Solid Edge part; units mm, degrees
sketch "Sketch1" plane through (0, 0, 0) normal (0, -1, 0) x (1, 0, 0)
  line L0 (-100, 125) -> (100, 125)
  line L1 (100, 125) -> (100, -125)
  line L2 (100, -125) -> (-100, -125)
  line L3 (-100, -125) -> (-100, 125)
  dimension "D1" = 100
  dimension "D2" = 100
extrude "Protrusion1" add sketch "Sketch1" along normal mid plane 6
sketch "Sketch2" plane through (0, -3, 0) normal (0, -1, 0) x (1, 0, 0)
  line L0 (-30, 55) -> (30, 55)
  line L1 (30, 55) -> (30, -5)
  line L2 (30, -5) -> (-30, -5)
  line L3 (-30, -5) -> (-30, 55)
  dimension "D1" = 30
  dimension "D2" = 30
extrude "Ausprägung_2" add sketch "Sketch2" along normal blind 1
hole "Bohrung_1" at (20, -4, 45) direction (0, 1, 0) diameter 8 end up to next
hole "Hole1" at (0, -4, 5) direction (0, 1, 0) diameter 8 end up to next
hole "Hole2" at (-20, -4, 45) direction (0, 1, 0) diameter 8 end up to next
sketch "Sketch3" plane through (0, -3, 0) normal (0, -1, 0) x (1, 0, 0)
  line L0 (-80, -125) -> (0, -45)
  line L1 (0, -45) -> (80, -125)
  line L2 (-80, -125) -> (80, -125)
  dimension "D1" = 80
extrude "Ausschnitt_1" cut sketch "Sketch3" against normal blind 146.05
sketch "Sketch4" plane through (0, -3, 0) normal (0, -1, 0) x (1, 0, 0)
  line L0 (-100, -105) -> (-30, -35)
  line L1 (-30, -35) -> (-30, -5)
  line L2 (-30, -5) -> (-30, 55)
  line L3 (-30, 55) -> (-100, 55)
  line L4 (-100, 55) -> (-100, -105)
  dimension "D1" = 100
extrude "Ausschnitt_2" cut sketch "Sketch4" against normal blind 200.025
sketch "Sketch5" plane through (0, -3, 0) normal (0, -1, 0) x (1, 0, 0)
  line L0 (100, -105) -> (30, -35)
  line L1 (30, -35) -> (30, -5)
  line L2 (30, -5) -> (30, 55)
  line L3 (30, 55) -> (100, 55)
  line L4 (100, 55) -> (100, -105)
extrude "Ausschnitt_3" cut sketch "Sketch5" against normal blind 184.15
sketch "Sketch6" plane through (0, -3, 90) normal (0, -1, 0) x (1, 0, 0)
  line L0 (-40, 35) -> (0, -5)
  line L1 (0, -5) -> (40, 35)
  line L2 (40, 35) -> (-40, 35)
  dimension "D1" = 40
extrude "Ausschnitt_4" cut sketch "Sketch6" against normal blind 88.9
sketch "Sketch7" plane through (0, -3, 90) normal (0, -1, 0) x (1, 0, 0)
  line L0 (-75.3553, 35) -> (-30, -10.3553)
  line L1 (-30, -10.3553) -> (-30, -35)
  line L2 (-30, -35) -> (-100, -35)
  line L3 (-100, -35) -> (-100, 35)
  line L4 (-100, 35) -> (-75.3553, 35)
  dimension "D1" = 30
extrude "Ausschnitt_5" cut sketch "Sketch7" against normal blind 38.1
sketch "Sketch8" plane through (12.3223, -3, 90) normal (0, -1, 0) x (1, 0, 0)
  line L0 (63.033, 35) -> (17.6777, -10.3553)
  line L1 (17.6777, -10.3553) -> (17.6777, -35)
  line L2 (17.6777, -35) -> (87.6777, -35)
  line L3 (87.6777, -35) -> (87.6777, 35)
  line L4 (87.6777, 35) -> (63.033, 35)
  dimension "D1" = 17.6777
extrude "Ausschnitt_6" cut sketch "Sketch8" against normal blind 104.775
sketch "Sketch9" plane through (0, -3, 90) normal (0, -1, 0) x (1, 0, 0)
  line L0 (-40, 35) -> (-57.6777, 17.3223)
  line L1 (-57.6777, 17.3223) -> (-75.3553, 35)
  line L2 (-75.3553, 35) -> (-40, 35)
extrude "Ausschnitt_7" cut sketch "Sketch9" against normal blind 63.5
sketch "Sketch10" plane through (8.8388, -3, 90) normal (0, -1, 0) x (1, 0, 0)
  line L0 (31.1612, 35) -> (48.8388, 17.3223)
  line L1 (48.8388, 17.3223) -> (66.5165, 35)
  line L2 (66.5165, 35) -> (31.1612, 35)
extrude "Ausschnitt_8" cut sketch "Sketch10" against normal blind 82.55
fillet "Verrundung_1" radius 12.5 4 edges at (-40, 0, 125) (-57.6777, 0, 107.3223) (40, 0, 125) (57.6777, 0, 107.3223)
sketch "Sketch11" plane through (0, -3, -65) normal (0, -1, 0) x (1, 0, 0)
  line L0 (-100, -40) -> (-80, -60)
  line L1 (-100, -40) -> (-100, -60)
  line L2 (-100, -60) -> (-80, -60)
extrude "Ausschnitt_9" cut sketch "Sketch11" against normal blind 60.325
sketch "Sketch12" plane through (-90, 0, -115) normal (-0.7071, 0, -0.7071) x (0, -1, 0)
  line L0 (-3, 14.1421) -> (3, 14.1421)
  line L1 (3, 14.1421) -> (3, -14.1421)
  line L2 (3, -14.1421) -> (-3, -14.1421)
  line L3 (-3, -14.1421) -> (-3, 14.1421)
extrude "Ausprägung_3" add sketch "Sketch12" along normal blind 14.14
sketch "Sketch13" plane through (-4.9992, -3, -69.9992) normal (0, -1, 0) x (-0.7071, 0, 0.7071)
  line L0 (-98.9949, -21.2121) -> (-98.9949, -49.4964)
  line L1 (-98.9949, -49.4964) -> (-113.1371, -35.3543)
  line L2 (-113.1371, -35.3543) -> (-98.9949, -21.2121)
extrude "Ausschnitt_10" cut sketch "Sketch13" against normal blind 63.5
sketch "Sketch14" plane through (90, 0, -115) normal (0.7071, 0, -0.7071) x (0.7071, 0, 0.7071)
  line L0 (-14.1421, 3) -> (14.1421, 3)
  line L1 (14.1421, 3) -> (14.1421, -3)
  line L2 (14.1421, -3) -> (-14.1421, -3)
  line L3 (-14.1421, -3) -> (-14.1421, 3)
extrude "Ausprägung_4" add sketch "Sketch14" along normal blind 14.14
fillet "Verrundung_2" radius 13.5 4 edges at (-109.9985, 0, -114.9985) (-89.9985, 0, -134.9985) (89.9985, 0, -134.9985) (109.9985, 0, -114.9985)
fillet "Verrundung_3" radius 5 6 edges at (-30, 0, -35) (-30, 0, 79.6447) (0, 0, 85) (30, 0, 79.6447) (30, 0, -35) (0, 0, -45)
properties material "Aluminium, 1060"
Part model, mm, in its own coordinate system. A direction names the side the tool comes from. Round coordinates to 2 decimals unless told otherwise and drop trailing zeros. Loops run counter-clockwise (first coordinate to the right, second up) from the corner with the lowest first, then second, coordinate; pieces in that order, holes last.
1. Slice it at C-C (z = 45). Give the cut face in (x, y), and give its area (3 significant figures).
Solutions:
outline: (-30, -4) - (-24, -4) - (-24, 3) - (-30, 3) - close; (-16, -4) - (16, -4) - (16, 3) - (-16, 3) - close; (24, -4) - (30, -4) - (30, 3) - (24, 3) - close
area: 308 mm2
2. 3-axis set-ups, long thin cutter, end or side, ignore diameter. For faces 1 (the face through (-30, -1, 23)), 2 (the face through (66, 0, -71)), 3 (the face through (16, -3, -54)), 4 (the face through (-42, 0, -87)): which of +Z, -Z, +X, -X, +Y, -Y reach the whole face in a straight line?
Solutions:
face 1: -X, +Y, -Y
face 2: +X, +Y, -Y
face 3: -Z, +X, -X, -Y
face 4: -Z, +Y, -Y
3. Drill centre lines: line 1 along X through (y, z) = (1.25, 45); line 2 along X through (y, z) = (1, 5); line 3 along Z through (x, y) = (0, -2). Where is each one in solid material? Low to high.
Solutions:
line 1: x = -30 to -24, -16 to 16, 24 to 30
line 2: x = -30 to -4, 4 to 30
line 3: z = -47.07 to 1, 9 to 87.07
4. Flat gauge pins, fed straight in: pin 1 (3 mm diameter, centred on y = -1, z = -35.5, fed in from -X); pin 2 (0.8 mm diameter, centred on x = 8, y = -3.5, fed in from -Z); pin 3 (3 mm diameter, centred on y = 1, z = 85.5, fed in from -X); pin 4 (13 mm diameter, centred on x = 20, z = 45, fed in from -Y). Where does each tip first touch, or does it go through?
Solutions:
pin 1: stops at x = -32
pin 2: stops at z = -5
pin 3: stops at x = -37.36
pin 4: stops at y = -4
5. Slice it at D-D (z = 5). Give the cut face in (x, y).
Solutions:
outline: (-30, -4) - (-4, -4) - (-4, 3) - (-30, 3) - close; (4, -4) - (30, -4) - (30, 3) - (4, 3) - close
6. Slice it at A-A (z = -59.5). Give the cut face in (x, y).
Solutions:
outline: (-54.5, -3) - (-14.5, -3) - (-14.5, 3) - (-54.5, 3) - close; (14.5, -3) - (54.5, -3) - (54.5, 3) - (14.5, 3) - close
7. Slice it at B-B (x = 20). Give the cut face in (y, z), and give its area (3 significant figures).
Solutions:
outline: (-4, -5) - (-3, -5) - (-3, -65) - (3, -65) - (3, 41) - (-4, 41) - close; (-4, 49) - (3, 49) - (3, 105) - (-3, 105) - (-3, 55) - (-4, 55) - close
area: 1,020 mm2
8. Two-plate mould, pull along Z, no slides. Class faces 5 (the face through (-40.137, 0.042, 119.822)), 6 (the face through (-17.3, -0.55, 47.95)), 7 (the face through (104.406, 0.042, -114.85)): pulls with the +Z half, pulls with the -Z half, needs draft (parallel to the pull), parting line crosses it, or undercut.
Solutions:
face 5: pulls with the +Z half
face 6: undercut
face 7: parting line crosses it
